Verification items for the finished model (mm, model axes). A direction names the side the tool comes from. Round coordinates to 2 decimals unless told otherwise and drop trailing zeros. Order: outer loops, then holes, each group sorted by start corner. A loop starts at its lowest first (then second) coordinate and runs counter-clockwise, first axis right, second up. Notation, with made-up numbers: (38, -25.75) -> (95, -25.75) arc R15 ccw to (95, -7.75) -> close; hole circle Ø3 at (42, 79). An arc over 180 degrees is marked (long way). Put each result on its own line as item: value.
```python
from build123d import *

# Parameters (mm, degrees)
SKETCH_1_W                       = 700
SKETCH_1_H                       = 580
EXTRUDE_1_DEPTH                  = 20
EXTRUDE_2_DEPTH                  = 12
CUT_EXTRUDE_1_REACH              = 521.038
SKETCH_3_R                       = 20
CUT_EXTRUDE_2_REACH              = 724.288
CUT_EXTRUDE_3_REACH              = 724.288
CUT_EXTRUDE_4_REACH              = 724.288
SKETCH_6_W                       = 100
SKETCH_6_H                       = 8
CUT_EXTRUDE_5_REACH              = 610.872
SKETCH_7_R                       = 2
CUT_EXTRUDE_6_REACH              = 610.872
SKETCH_8_R                       = 2
PATTERN_LINEAR_1_COUNT           = 5
PATTERN_LINEAR_1_PITCH           = 20
CUT_EXTRUDE_7_REACH              = 724.288
SKETCH_9_W                       = 131
SKETCH_9_H                       = 8
SKETCH_13_R                      = 5.5
CUT_EXTRUDE_10_DEPTH             = 5
PATTERN_LINEAR_2_COUNT           = 2
PATTERN_LINEAR_2_PITCH           = 300
PATTERN_LINEAR_3_COUNT           = 2
PATTERN_LINEAR_3_PITCH           = 325
PATTERN_LINEAR_3_COPY_1_SKETCH_R = 5.5
PATTERN_LINEAR_3_COPY_1_DEPTH    = 5
SKETCH_15_W                      = 80
SKETCH_15_H                      = 80
EXTRUDE_3_DEPTH                  = 3
SKETCH_16_R                      = 9.25
CUT_EXTRUDE_11_DEPTH             = 520.16212535
SKETCH_15_3_R                    = 9.25
CUT_EXTRUDE_12_DEPTH             = 15


with BuildPart() as part:
    # Sketch 1 → Extrude 1 (new body)
    with BuildSketch(Plane(origin=(0, 0, 0), x_dir=(1, 0, 0), z_dir=(0, 1, 0))):
        Rectangle(SKETCH_1_W, SKETCH_1_H)
    extrude(amount=EXTRUDE_1_DEPTH)

    # Sketch 2 → Extrude 2 (add)
    with BuildSketch(Plane(origin=(0, 20, 0), x_dir=(1, 0, 0), z_dir=(0, 1, 0))):
        Polygon((350, -135.000538617), (350, -290), (430, -290.000538617), (430, -135.000538617), align=None)
    extrude(amount=-EXTRUDE_2_DEPTH)

    # Sketch 3 → Cut-Extrude 1 (cut, up to next)
    with BuildSketch(Plane(origin=(0, 20, 0), x_dir=(1, 0, 0), z_dir=(0, 1, 0)), mode=Mode.PRIVATE) as cut_extrude_1_sk1:
        with Locations(Location((390, -212.500538617, 0), (0, 0, 270))):
            Circle(SKETCH_3_R)
    cut_extrude_1_tool1 = extrude(cut_extrude_1_sk1.sketch, amount=-CUT_EXTRUDE_1_REACH, mode=Mode.PRIVATE) & part.part
    add(cut_extrude_1_tool1.solids().sort_by_distance((390, 20, 212.500539))[0], mode=Mode.SUBTRACT)

    # Sketch 4 → Cut-Extrude 2 (cut, up to next)
    with BuildSketch(Plane(origin=(0, 0, -290), x_dir=(-1, 0, 0), z_dir=(0, 0, -1)), mode=Mode.PRIVATE) as cut_extrude_2_sk1:
        Polygon((-170, 0), (-170, 8), (-170, 11), (-165, 11), (-165, 8), (-46.060660172, 8), (-45.353553391, 8.707106781), (-44.292893219, 7.646446609), (-45, 6.939339828), (-45, 0), align=None)
    cut_extrude_2_tool1 = extrude(cut_extrude_2_sk1.sketch, amount=-CUT_EXTRUDE_2_REACH, mode=Mode.PRIVATE) & part.part
    add(cut_extrude_2_tool1.solids().sort_by_distance((108.328272, 4.084832, -290))[0], mode=Mode.SUBTRACT)

    # Sketch 5 → Cut-Extrude 3 (cut, up to next)
    with BuildSketch(Plane(origin=(0, 0, -290), x_dir=(-1, 0, 0), z_dir=(0, 0, -1)), mode=Mode.PRIVATE) as cut_extrude_3_sk1:
        Polygon((-5, 0), (-5, 10), (135, 10), (137, 8), (350, 8), (350, 0), (167, 0), align=None)
    cut_extrude_3_tool1 = extrude(cut_extrude_3_sk1.sketch, amount=-CUT_EXTRUDE_3_REACH, mode=Mode.PRIVATE) & part.part
    add(cut_extrude_3_tool1.solids().sort_by_distance((-162.835148, 4.45142, -290))[0], mode=Mode.SUBTRACT)

    # Sketch 6 → Cut-Extrude 4 (cut, up to next)
    with BuildSketch(Plane(origin=(0, 0, -290), x_dir=(-1, 0, 0), z_dir=(0, 0, -1)), mode=Mode.PRIVATE) as cut_extrude_4_sk1:
        with Locations((-235, 4)):
            Rectangle(SKETCH_6_W, SKETCH_6_H)
    cut_extrude_4_tool1 = extrude(cut_extrude_4_sk1.sketch, amount=-CUT_EXTRUDE_4_REACH, mode=Mode.PRIVATE) & part.part
    add(cut_extrude_4_tool1.solids().sort_by_distance((235, 4, -290))[0], mode=Mode.SUBTRACT)

    # Sketch 7 → Cut-Extrude 5 (cut, up to next)
    with BuildSketch(Plane(origin=(185, 0, 0), x_dir=(0, 0, -1), z_dir=(1, 0, 0)), mode=Mode.PRIVATE) as cut_extrude_5_sk1:
        with Locations((200, 4)):
            Circle(SKETCH_7_R)
    cut_extrude_5_tool1 = extrude(cut_extrude_5_sk1.sketch, amount=-CUT_EXTRUDE_5_REACH, mode=Mode.PRIVATE) & part.part
    # Sketch 7 → Cut-Extrude 5 (cut, up to next)
    with BuildSketch(Plane(origin=(185, 0, 0), x_dir=(0, 0, -1), z_dir=(1, 0, 0)), mode=Mode.PRIVATE) as cut_extrude_5_sk2:
        with Locations((180, 4)):
            Circle(SKETCH_7_R)
    cut_extrude_5_tool2 = extrude(cut_extrude_5_sk2.sketch, amount=-CUT_EXTRUDE_5_REACH, mode=Mode.PRIVATE) & part.part
    # Sketch 7 → Cut-Extrude 5 (cut, up to next)
    with BuildSketch(Plane(origin=(185, 0, 0), x_dir=(0, 0, -1), z_dir=(1, 0, 0)), mode=Mode.PRIVATE) as cut_extrude_5_sk3:
        with Locations((160, 4)):
            Circle(SKETCH_7_R)
    cut_extrude_5_tool3 = extrude(cut_extrude_5_sk3.sketch, amount=-CUT_EXTRUDE_5_REACH, mode=Mode.PRIVATE) & part.part
    # Sketch 7 → Cut-Extrude 5 (cut, up to next)
    with BuildSketch(Plane(origin=(185, 0, 0), x_dir=(0, 0, -1), z_dir=(1, 0, 0)), mode=Mode.PRIVATE) as cut_extrude_5_sk4:
        with Locations((140, 4)):
            Circle(SKETCH_7_R)
    cut_extrude_5_tool4 = extrude(cut_extrude_5_sk4.sketch, amount=-CUT_EXTRUDE_5_REACH, mode=Mode.PRIVATE) & part.part
    # Sketch 7 → Cut-Extrude 5 (cut, up to next)
    with BuildSketch(Plane(origin=(185, 0, 0), x_dir=(0, 0, -1), z_dir=(1, 0, 0)), mode=Mode.PRIVATE) as cut_extrude_5_sk5:
        with Locations((120, 4)):
            Circle(SKETCH_7_R)
    cut_extrude_5_tool5 = extrude(cut_extrude_5_sk5.sketch, amount=-CUT_EXTRUDE_5_REACH, mode=Mode.PRIVATE) & part.part
    add(cut_extrude_5_tool1.solids().sort_by_distance((185, 4, -200))[0], mode=Mode.SUBTRACT)
    add(cut_extrude_5_tool2.solids().sort_by_distance((185, 4, -180))[0], mode=Mode.SUBTRACT)
    add(cut_extrude_5_tool3.solids().sort_by_distance((185, 4, -160))[0], mode=Mode.SUBTRACT)
    add(cut_extrude_5_tool4.solids().sort_by_distance((185, 4, -140))[0], mode=Mode.SUBTRACT)
    add(cut_extrude_5_tool5.solids().sort_by_distance((185, 4, -120))[0], mode=Mode.SUBTRACT)

    # Sketch 8 → Cut-Extrude 6 (cut, up to next)
    with BuildSketch(Plane(origin=(185, 0, 0), x_dir=(0, 0, -1), z_dir=(1, 0, 0)), mode=Mode.PRIVATE) as cut_extrude_6_sk1:
        with Locations((-125, 4)):
            Circle(SKETCH_8_R)
    cut_extrude_6_tool1 = extrude(cut_extrude_6_sk1.sketch, amount=-CUT_EXTRUDE_6_REACH, mode=Mode.PRIVATE) & part.part
    cut_extrude_6 = cut_extrude_6_tool1.solids().sort_by_distance((185, 4, 125))[0]
    add(cut_extrude_6, mode=Mode.SUBTRACT)

    # Pattern Linear 1: Cut-Extrude 6 ×5
    with Locations(*[(0, 0, i * PATTERN_LINEAR_1_PITCH) for i in range(1, PATTERN_LINEAR_1_COUNT)]):
        add(cut_extrude_6, mode=Mode.SUBTRACT)

    # Sketch 9 → Cut-Extrude 7 (cut, up to next)
    with BuildSketch(Plane.XY.offset(290), mode=Mode.PRIVATE) as cut_extrude_7_sk1:
        with Locations((364.5, 4)):
            Rectangle(SKETCH_9_W, SKETCH_9_H)
    cut_extrude_7_tool1 = extrude(cut_extrude_7_sk1.sketch, amount=-CUT_EXTRUDE_7_REACH, mode=Mode.PRIVATE) & part.part
    add(cut_extrude_7_tool1.solids().sort_by_distance((364.5, 4, 290))[0], mode=Mode.SUBTRACT)

    # Sketch 13 → Cut-Extrude 10 (cut)
    with BuildSketch(Plane.XZ.offset(-8)):
        with Locations(Location((-245, 137.5, 0), (0, 0, 270))):
            Circle(SKETCH_13_R)
        with Locations(Location((-245, 197.5, 0), (0, 0, 270))):
            Circle(SKETCH_13_R)
        with Locations(Location((-145, 197.5, 0), (0, 0, 270))):
            Circle(SKETCH_13_R)
        with Locations(Location((-145, 137.5, 0), (0, 0, 270))):
            Circle(SKETCH_13_R)
    cut_extrude_10 = extrude(amount=-CUT_EXTRUDE_10_DEPTH, mode=Mode.SUBTRACT)

    # Pattern Linear 2: Cut-Extrude 10 ×2
    with Locations(*[(i * PATTERN_LINEAR_2_PITCH, 0, 0) for i in range(1, PATTERN_LINEAR_2_COUNT)]):
        add(cut_extrude_10, mode=Mode.SUBTRACT)

    # Pattern Linear 3: Cut-Extrude 10 ×2
    with Locations(*[(0, 0, -i * PATTERN_LINEAR_3_PITCH) for i in range(1, PATTERN_LINEAR_3_COUNT)]):
        add(cut_extrude_10, mode=Mode.SUBTRACT)

    # Pattern Linear 3 copy 1 sketch → Pattern Linear 3 copy 1 (cut)
    with BuildSketch(Plane(origin=(300, 8, -325), x_dir=(1, 0, 0), z_dir=(0, -1, 0))):
        with Locations(Location((-245, 137.5, 0), (0, 0, 270))):
            Circle(PATTERN_LINEAR_3_COPY_1_SKETCH_R)
        with Locations(Location((-245, 197.5, 0), (0, 0, 270))):
            Circle(PATTERN_LINEAR_3_COPY_1_SKETCH_R)
        with Locations(Location((-145, 197.5, 0), (0, 0, 270))):
            Circle(PATTERN_LINEAR_3_COPY_1_SKETCH_R)
        with Locations(Location((-145, 137.5, 0), (0, 0, 270))):
            Circle(PATTERN_LINEAR_3_COPY_1_SKETCH_R)
    extrude(amount=-PATTERN_LINEAR_3_COPY_1_DEPTH, mode=Mode.SUBTRACT)

    # Sketch 15 → Extrude 3 (add)
    with BuildSketch(Plane(origin=(0, 20, 0), x_dir=(1, 0, 0), z_dir=(0, 1, 0))):
        with Locations((72, -215)):
            Rectangle(SKETCH_15_W, SKETCH_15_H)
        with Locations((72, 215)):
            Rectangle(SKETCH_15_W, SKETCH_15_H)
        with Locations((-301.459594093, 4.399478147)):
            Rectangle(SKETCH_15_W, SKETCH_15_H)
    extrude(amount=EXTRUDE_3_DEPTH)

    # Sketch 16 → Cut-Extrude 11 (cut, through all)
    with BuildSketch(Plane(origin=(0, 23, 0), x_dir=(1, 0, 0), z_dir=(0, 1, 0))):
        with Locations(Location((-301.914277382, 0.259141217, 0), (0, 0, 270))):
            Circle(SKETCH_16_R)
    extrude(amount=-CUT_EXTRUDE_11_DEPTH, mode=Mode.SUBTRACT)

    # Sketch 15_3 → Cut-Extrude 12 (cut, symmetric)
    with BuildSketch(Plane(origin=(0, 20, 0), x_dir=(1, 0, 0), z_dir=(0, 1, 0))):
        with Locations(Location((73.085716832, -216.247219752, 0), (0, 0, 270))):
            Circle(SKETCH_15_3_R)
        with Locations(Location((73.085716832, 216.247219752, 0), (0, 0, 270))):
            Circle(SKETCH_15_3_R)
    extrude(amount=CUT_EXTRUDE_12_DEPTH, both=True, mode=Mode.SUBTRACT)


solid = part.part
```
Item 1: Material ranges on line 1 along X through (y, z) = (6.25, -103); line 2 along X through (y, z) = (8.25, -102.5); line 3 along X through (y, z) = (2.5, -179), recorded low to high.
Geometry check:
line 1: 5 to 45, 170 to 185, 285 to 299
line 2: -350 to -136.75, 5 to 44.9, 45.81 to 165, 170 to 350
line 3: 5 to 45, 285 to 299
Item 2: Sectioned sample at B-B, the plane z = -70.5. Record the boundary of the cut face in (x, y).
Geometry check:
outline: (-350, 8) -> (-137, 8) -> (-135, 10) -> (5, 10) -> (5, 0) -> (45, 0) -> (45, 6.94) -> (44.29, 7.65) -> (45.35, 8.71) -> (46.06, 8) -> (165, 8) -> (165, 11) -> (170, 11) -> (170, 0) -> (185, 0) -> (185, 8) -> (285, 8) -> (285, 0) -> (299, 0) -> (299, 8) -> (350, 8) -> (350, 20) -> (-350, 20) -> close
Item 3: Tool access check on faces 4 (the face through (106, 8, -4)), 5 (the face through (334, 8, 60)), 6 (the face through (-242, 8, -4)). Record the directions out of +Z, -Z, +X, -X, +Y, -Y that give a thin tool (end or side, any length) a straight path to the whole face; none if there is none.
Geometry check:
face 4: +Z, -Z, -Y
face 5: +Z, -Z, +X, -Y
face 6: +Z, -Z, -X, -Y
Item 4: Depth check by flat-ended pin: pin 1 Ø9 at (y, z) = (6, 25) entering from +X; pin 2 Ø9 at (x, z) = (-242.5, -130) entering from -Y; pin 3 Ø11 at (y, z) = (4.5, -68) entering from -X; pin 4 Ø12.5 at (x, z) = (-245, 137.5) entering from +Y. Enter the tip coordinate at first touch or a pass-through.
Geometry check:
pin 1: x = 350
pin 2: y = 8
pin 3: x = -350
pin 4: y = 20
Item 5: Release check for a two-part mould opening along Z. For faces 1 (the face through (75.864, 15.605, -207.424)), 2 (the face through (-5, 14, -290)), 3 (the face through (236, 8, -4)) record: pulls with the +Z half, pulls with the -Z half, needs draft (parallel to the pull), parting line crosses it, or undercut.
Geometry check:
face 1: undercut
face 2: pulls with the -Z half
face 3: needs draft
Item 6: Sectioned sample at A-A, the plane z = 25. Record the boundary of the cut face in (x, y), then the cut area to 3 significant figures.
Geometry check:
outline: (-350, 8) -> (-137, 8) -> (-135, 10) -> (5, 10) -> (5, 0) -> (45, 0) -> (45, 6.94) -> (44.29, 7.65) -> (45.35, 8.71) -> (46.06, 8) -> (165, 8) -> (165, 11) -> (170, 11) -> (170, 0) -> (185, 0) -> (185, 8) -> (285, 8) -> (285, 0) -> (299, 0) -> (299, 8) -> (350, 8) -> (350, 20) -> (-261.46, 20) -> (-261.46, 23) -> (-341.46, 23) -> (-341.46, 20) -> (-350, 20) -> close
area: 8,890 mm2
